```python
from build123d import *

# Parameters (mm, degrees)
SKETCH_1_R      = 28.5
SKETCH_1_R_2    = 2.5
SKETCH_1_R_3    = 18
SKETCH_1_R_4    = 11
EXTRUDE_3_DEPTH = 3
SKETCH_3_R      = 18
SKETCH_3_R_2    = 11
SKETCH_3_R_3    = 2.5
EXTRUDE_4_DEPTH = 8


with BuildPart() as part:
    # 草图1 → 凸台-拉伸3 (new body)
    # profile 1 of 2: a face of its own
    with BuildSketch(Plane.XY):
        Circle(SKETCH_1_R)
        with Locations((-12.5, -21.650635095)):
            Circle(SKETCH_1_R_2, mode=Mode.SUBTRACT)
        with Locations((12.5, -21.650635095)):
            Circle(SKETCH_1_R_2, mode=Mode.SUBTRACT)
        with Locations((25, 0)):
            Circle(SKETCH_1_R_2, mode=Mode.SUBTRACT)
        with Locations((12.846045577, 21.051266574)):
            Circle(SKETCH_1_R_2, mode=Mode.SUBTRACT)
        with Locations((-25, 0)):
            Circle(SKETCH_1_R_2, mode=Mode.SUBTRACT)
        with Locations((-12.5, 21.650635095)):
            Circle(SKETCH_1_R_2, mode=Mode.SUBTRACT)
        Circle(SKETCH_1_R_3, mode=Mode.SUBTRACT)
    # profile 2 of 2: a face of its own
    with BuildSketch(Plane.XY):
        Circle(SKETCH_1_R_3)
        Circle(SKETCH_1_R_4, mode=Mode.SUBTRACT)
        with Locations((-7.25, 12.557368355)):
            Circle(SKETCH_1_R_2, mode=Mode.SUBTRACT)
        with Locations((7.25, 12.557368355)):
            Circle(SKETCH_1_R_2, mode=Mode.SUBTRACT)
        with Locations((-14.5, 0)):
            Circle(SKETCH_1_R_2, mode=Mode.SUBTRACT)
        with Locations((14.5, 0)):
            Circle(SKETCH_1_R_2, mode=Mode.SUBTRACT)
        with Locations((7.25, -12.557368355)):
            Circle(SKETCH_1_R_2, mode=Mode.SUBTRACT)
        with Locations((-7.25, -12.557368355)):
            Circle(SKETCH_1_R_2, mode=Mode.SUBTRACT)
    extrude(amount=EXTRUDE_3_DEPTH)

    # 草图3 → 凸台-拉伸4 (add)
    with BuildSketch(Plane.XY.offset(3)):
        Circle(SKETCH_3_R)
        Circle(SKETCH_3_R_2, mode=Mode.SUBTRACT)
        with Locations((-14.5, 0)):
            Circle(SKETCH_3_R_3, mode=Mode.SUBTRACT)
        with Locations((-7.25, 12.557368355)):
            Circle(SKETCH_3_R_3, mode=Mode.SUBTRACT)
        with Locations((7.25, 12.557368355)):
            Circle(SKETCH_3_R_3, mode=Mode.SUBTRACT)
        with Locations((14.5, 0)):
            Circle(SKETCH_3_R_3, mode=Mode.SUBTRACT)
        with Locations((7.25, -12.557368355)):
            Circle(SKETCH_3_R_3, mode=Mode.SUBTRACT)
        with Locations((-7.25, -12.557368355)):
            Circle(SKETCH_3_R_3, mode=Mode.SUBTRACT)
    extrude(amount=EXTRUDE_4_DEPTH)


solid = part.part
```
Work out the finished part from the listing and answer in its coordinate system (mm). A direction names the side the tool comes from. Give positions to 0.01 mm unless a question says otherwise; leave off trailing zeros. Write each loop counter-clockwise with the first axis right and the second up, starting at its lowest first coordinate (ties: lowest second). Pieces come first, ordered by that corner, then holes. Notation, with made-up numbers: (-9, -22.75) -> (45, -22.75) arc R21 cw to (45, -5.75) -> close; hole circle Ø3 at (45, 30.5). An arc over 180 degrees is marked (long way). Write each question's results on one line, items separated by ' | '.
1. Straight lines are drawn through the part: L1, parallel to Y at x = -5, z = 2; L2, parallel to Y at x = 7.25, z = 6.25; L3, parallel to X at y = 20, z = 2. For each, find the intervals that lie inside material, in ascending order.
Data:
L1: -28.06 to -13.65, -11.47 to -9.8, 9.8 to 11.47, 13.65 to 28.06 | L2: -16.48 to -15.06, -10.06 to -8.27, 8.27 to 10.06, 15.06 to 16.48 | L3: -20.3 to -14.38, -10.62 to 10.58, 15.11 to 20.3
2. Find section B-B on y = -22.5. Determine the outline of the cut face in (x, z).
Data:
outline: (-17.49, 0) -> (-14.85, 0) -> (-14.85, 3) -> (-17.49, 3) -> close; (-10.15, 0) -> (10.15, 0) -> (10.15, 3) -> (-10.15, 3) -> close; (14.85, 0) -> (17.49, 0) -> (17.49, 3) -> (14.85, 3) -> close
3. Determine the mould class of faces 3 (the flat face through (11.7, 0.3, 11)), 4 (the cylindrical face through (-27.5, 0.1, 1.5)), 5 (the cylindrical face through (-2.343, 17.847, 6.944)) for opening direction Y: +Y half, -Y half, draft (parallel to the pull), parting line (faces both ways), or undercut.
Data:
face 3: draft | face 4: undercut | face 5: parting line
4. Find section D-D on z = 1.25. Give the number of separate pieces and of enclosed holes in the cut face, and give its area (3 significant figures).
Data:
separate pieces: 1 | enclosed holes: 13 | area: 1,940 mm^2
5. Find section A-A on y = 0. Determine the outline of the cut face in (x, z), and give its area (3 significant figures).
Data:
outline: (-28.5, 0) -> (-27.5, 0) -> (-27.5, 3) -> (-28.5, 3) -> close; (-22.5, 0) -> (-17, 0) -> (-17, 11) -> (-18, 11) -> (-18, 3) -> (-22.5, 3) -> close; (-12, 0) -> (-11, 0) -> (-11, 11) -> (-12, 11) -> close; (11, 0) -> (12, 0) -> (12, 11) -> (11, 11) -> close; (17, 0) -> (22.5, 0) -> (22.5, 3) -> (18, 3) -> (18, 11) -> (17, 11) -> close; (27.5, 0) -> (28.5, 0) -> (28.5, 3) -> (27.5, 3) -> close | area: 77.0 mm^2
6. Each of these flat-tipped pins is pushed along its axis until it touches: pin 1 Ø6 at (x, y) = (7.25, -12.56) entering from +Z; pin 2 Ø6.5 at (x, y) = (-12.5, -21.65) entering from +Z; pin 3 Ø1.5 at (y, z) = (13.5, 7.5) entering from -X; pin 4 Ø1.5 at (y, z) = (13.5, 2) entering from +X. Where does it stop, or does it pass through?
Data:
pin 1: z = 11 | pin 2: z = 3 | pin 3: x = -12.71 | pin 4: x = 25.49
7. A tool of negligible diameter and unlimited length cuts with its end or side. For faces 1 (the flat face through (0, -19, 3)), 2 (the cylindrical face through (-17, 0, 5)), from which of +Z, -Z, +X, -X, +Y, -Y can it reach the whole face along a straight path? Write none if from no direction.
Data:
face 1: +Z | face 2: +Z, -Z
8. Find section C-C on x = 9. Determine the outline of the cut face in (y, z), and give its area (3 significant figures).
Data:
outline: (-27.04, 0) -> (-14.34, 0) -> (-14.34, 11) -> (-15.59, 11) -> (-15.59, 3) -> (-27.04, 3) -> close; (-10.77, 0) -> (-6.32, 0) -> (-6.32, 11) -> (-10.77, 11) -> close; (6.32, 0) -> (10.77, 0) -> (10.77, 11) -> (6.32, 11) -> close; (14.34, 0) -> (27.04, 0) -> (27.04, 3) -> (15.59, 3) -> (15.59, 11) -> (14.34, 11) -> close | area: 194 mm^2
